Geometry: see drawing. Coordinates: mm, zero at the bounding-box minimum. A direction names the side the tool comes from. Coordinates: 2 decimals unless noted, no trailing zeros. Order: outer loops, then holes, each group sorted by start corner. A loop starts at its lowest first (then second) coordinate and runs counter-clockwise, first axis right, second up. Notation, with made-up numbers: (61, 69) -> (85, 69) arc R21 cw to (85, 104) -> close; hole circle Ø8 at (-12, 13.25). An arc over 180 degrees is marked (long way). Write each question's results on one line, items separated by ' | '.
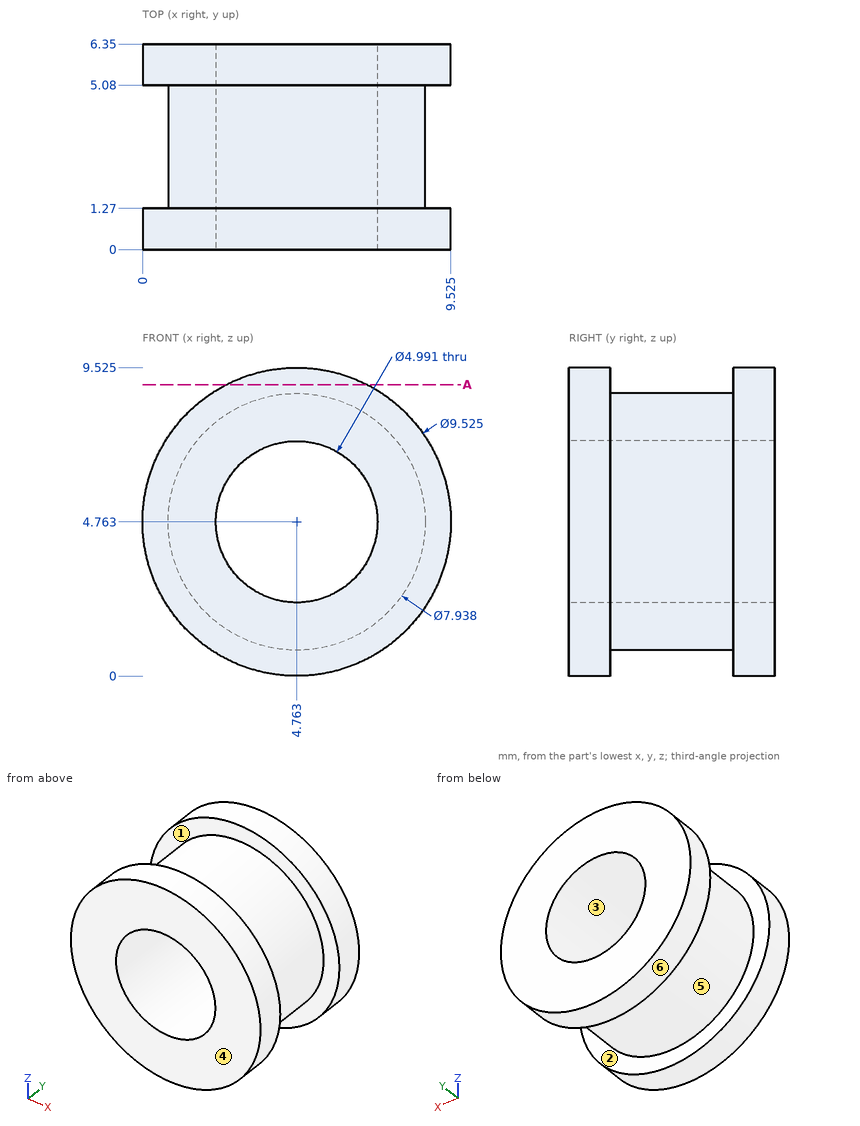
(1) Cut plane A-A, the plane z = 9. Return loops of the section in (x, y).
Return value:
outline: (2.59, 0) -> (6.94, 0) -> (6.94, 1.27) -> (2.59, 1.27) -> close; (2.59, 5.08) -> (6.94, 5.08) -> (6.94, 6.35) -> (2.59, 6.35) -> close
(2) Pin query (flat end, axial travel): P1, Ø1, axis at y = 2.5, z = 5.5, coming from the -X side; P2, Ø2, axis at x = 7, y = 2, coming from the +Z side (1 decimal). Return the tip coordinate at first contact, or that it passes through.
Return value:
P1: x = 0.8 | P2: z = 9.3
(3) Mould query, pull axis Y, two halves, no side actions, for the marked faces 1, 2, 3 and 4. Classes: +Y half, -Y half, draft (parallel to the pull), parting line (faces both ways), or undercut.
Return value:
face 1: undercut | face 2: undercut | face 3: draft | face 4: -Y half
(4) Line query: line 1 along Y through (x, z) = (1, 2.75); line 2 along Z through (x, y) = (2.5, 2.25) (1 decimal); line 3 along X through (y, z) = (3, 4.5) (1 decimal). Output: solid intervals per line, ascending. Write a range as from..to.
Return value:
line 1: 0..1.27, 5.08..6.35 | line 2: 1.5..3.7, 5.8..8 | line 3: 0.8..2.3, 7.2..8.7
(5) Reachability of the marked faces 5 and 6 from +Z, -Z, +X, -X, +Y, -Y: full face, straight path, thin tool, end or side. Return the list, or none.
Return value:
face 5: none | face 6: +Y, -Y
